from build123d import *

# Parameters (mm, degrees)
SKETCH1_R           = 2.5
BOSS_EXTRUDE2_DEPTH = 4


with BuildPart() as part:
    # Sketch1 → Boss-Extrude2 (new body)
    with BuildSketch(Plane(origin=(0, 0, 0), x_dir=(1, 0, 0), z_dir=(0, 1, 0))):
        with BuildLine():
            Line((-50, -27), (-50, 77))
            ThreePointArc((-50, 77), (-43.263455967, 93.263455967), (-27, 100))
            Line((-27, 100), (27, 100))
            ThreePointArc((27, 100), (43.263455967, 93.263455967), (50, 77))
            Line((50, 77), (50, -27))
            ThreePointArc((50, -27), (43.263455967, -43.263455967), (27, -50))
            Line((27, -50), (-27, -50))
            ThreePointArc((-27, -50), (-43.263455967, -43.263455967), (-50, -27))
        make_face()
        with Locations((-36, -36)):
            Circle(SKETCH1_R, mode=Mode.SUBTRACT)
        with Locations((-36, 86)):
            Circle(SKETCH1_R, mode=Mode.SUBTRACT)
        with Locations((36, -36)):
            Circle(SKETCH1_R, mode=Mode.SUBTRACT)
        with Locations((36, 86)):
            Circle(SKETCH1_R, mode=Mode.SUBTRACT)
        with BuildLine():
            Line((-27, -30), (27, -30))
            ThreePointArc((27, -30), (29.121320344, -29.121320344), (30, -27))
            Line((30, -27), (30, 27))
            ThreePointArc((30, 27), (29.121320344, 29.121320344), (27, 30))
            Line((27, 30), (20.5, 30))
            ThreePointArc((20.5, 30), (18.378679656, 30.878679656), (17.5, 33))
            Line((17.5, 33), (17.5, 77))
            ThreePointArc((17.5, 77), (16.621320344, 79.121320344), (14.5, 80))
            Line((14.5, 80), (-14.5, 80))
            ThreePointArc((-14.5, 80), (-16.621320344, 79.121320344), (-17.5, 77))
            Line((-17.5, 77), (-17.5, 33))
            ThreePointArc((-17.5, 33), (-18.378679656, 30.878679656), (-20.5, 30))
            Line((-20.5, 30), (-27, 30))
            ThreePointArc((-27, 30), (-29.121320344, 29.121320344), (-30, 27))
            Line((-30, 27), (-30, -27))
            ThreePointArc((-30, -27), (-29.121320344, -29.121320344), (-27, -30))
        make_face(mode=Mode.SUBTRACT)
    extrude(amount=BOSS_EXTRUDE2_DEPTH)


solid = part.part
Could you check a few things on this model? Use its own coordinates, in mm. A direction names the side the tool comes from. Coordinates: 2 decimals unless noted, no trailing zeros. Order: outer loops, then holes, each group sorted by start corner. A loop starts at its lowest first (then second) coordinate and runs counter-clockwise, first axis right, second up.
Q1. Which directions (+Z, -Z, +X, -X, +Y, -Y) give clear straight access to the entire face, cutting with the end or side of a thin tool? Please do faces 1 (the cylindrical face through (-29.14, 1.97, 29.1)), 2 (the cylindrical face through (43.441, 1.972, 43.084)).
Q2. Please list where these lines run through material, in increasing order: L1, parallel to Z at x = -1.5, y = 3.3; L2, parallel to X at y = 2, z = -86; L3, parallel to Z at x = 36, y = 1.2.
Q3. Suppose I cut it at C-C on y = 2.3. Please give me the cut outline in (x, z).
Q4. Suppose I cut it at A-A on z = -0.5. Please give me the cut outline in (x, y), and give its area (3 significant figures).
Q5. Suppose I cut it at B-B on x = -9. Please give me the cut outline in (y, z), and give its area (3 significant figures).
Q6. Will this pin go through, and if not, where does the flat tip stop? pin 1 (10 mm diameter, centred on x = -4.5, z = -79.5, fed in from +Y).
Q7. Suppose I cut it at D-D on x = -36. Please give me the cut outline in (y, z), and give its area (3 significant figures).
Q8. Thinking about a two-plate mould opening in Z: for faces 3 (the cylindrical face through (18.4, 1.97, -30.86)), 4 (the flat face through (-22, 4, -43)), 5 (the flat face through (0, 2, -100)), 6 (the cylindrical face through (16.64, 1.97, -79.1)), which applies, released by +Z, released by -Z, zero draft, split by the parting line, or undercut?
Answer:
1. face 1: +Y, -Y
1. face 2: +Z, +X, +Y, -Y
2. L1: z = -100 to -80, 30 to 50
2. L2: x = -48.17 to -38.5, -33.5 to 33.5, 38.5 to 48.17
2. L3: z = -98.17 to -88.5, -83.5 to 33.5, 38.5 to 48.17
3. outline: (-50, -77) arc R23 ccw to (-27, -100) - (27, -100) arc R23 ccw to (50, -77) - (50, 27) arc R23 ccw to (27, 50) - (-27, 50) arc R23 ccw to (-50, 27) - close; hole circle Ø5 at (-36, -86); hole circle Ø5 at (-36, 36); hole (-30, -27) arc R3 ccw to (-27, -30) - (-20.5, -30) arc R3 cw to (-17.5, -33) - (-17.5, -77) arc R3 ccw to (-14.5, -80) - (14.5, -80) arc R3 ccw to (17.5, -77) - (17.5, -33) arc R3 cw to (20.5, -30) - (27, -30) arc R3 ccw to (30, -27) - (30, 27) arc R3 ccw to (27, 30) - (-27, 30) arc R3 ccw to (-30, 27) - close; hole circle Ø5 at (36, -86); hole circle Ø5 at (36, 36)
4. outline: (-50, 0) - (-30, 0) - (-30, 4) - (-50, 4) - close; (30, 0) - (50, 0) - (50, 4) - (30, 4) - close
4. area: 160 mm2
5. outline: (0, -100) - (4, -100) - (4, -80) - (0, -80) - close; (0, 30) - (4, 30) - (4, 50) - (0, 50) - close
5. area: 160 mm2
6. pin 1: stops at y = 4
7. outline: (0, -98.17) - (4, -98.17) - (4, -88.5) - (0, -88.5) - close; (0, -83.5) - (4, -83.5) - (4, 33.5) - (0, 33.5) - close; (0, 38.5) - (4, 38.5) - (4, 48.17) - (0, 48.17) - close
7. area: 545 mm2
8. face 3: undercut
8. face 4: zero draft
8. face 5: released by -Z
8. face 6: undercut
